Could you check a few things on this model? Use its own coordinates, in mm. A direction names the side the tool comes from. Give positions to 0.01 mm unless a question says otherwise; leave off trailing zeros. Write each loop counter-clockwise with the first axis right and the second up, starting at its lowest first coordinate (ties: lowest second). Pieces come first, ordered by that corner, then holes. Notation, with made-up numbers: (3, -14.75) -> (16, -14.75) arc R18 ccw to (16, 11.25) -> close; hole circle Ø10 at (-18, 57). An arc over 180 degrees is marked (long way). One line per question, with ' | ' between items.
from build123d import *

# Parameters (mm, degrees)
F0_R     = 6.5
F1_DEPTH = 2.5
F3_DEPTH = 9.6


# Not quite as in the source:
# - a feature of the source that left no trace in its solid (it failed there, or was rolled back) is left out


with BuildPart() as f1:
    # F0 (on Top) → F1 (new body)
    with BuildSketch(Plane.XY):
        Polygon((-30.6198447943, 27.4039022624), (-27.4521095872, 27.4039022624), (-8.6198447943, 27.4039022624), (-8.6198447943, 35.4039022624), (-13.1198447943, 35.4039022624), (-13.1198447943, 42.8039022624), (-22.6198447943, 42.8039022624), (-22.6198447943, 46.4039022624), (-30.6198447943, 46.4039022624), align=None)
        Polygon((-3.2843746781, 35.4039022624), (-3.2843746781, 27.4039022624), (15.5478901148, 27.4039022624), (18.7156253219, 27.4039022624), (18.7156253219, 46.4039022624), (10.7156253219, 46.4039022624), (10.7156253219, 42.8039022624), (1.2156253219, 42.8039022624), (1.2156253219, 35.4039022624), align=None)
        Polygon((-8.6198447943, 27.4039022624), (-27.4521095872, 27.4039022624), (-27.4521095872, -26.3960977376), (-6.0521095872, -26.3960977376), (-5.8521098852, -26.3960977376), (15.5478901148, -26.3960977376), (15.5478901148, 27.4039022624), (-3.2843746781, 27.4039022624), (-5.8521098852, 27.4039022624), (-6.0521095872, 27.4039022624), align=None)
        Polygon((-23.4521095872, -22.3960977376), (-23.4521095872, 23.4039022624), (-5.9521097362, 23.4039022624), (11.5478901148, 23.4039022624), (11.5478901148, -22.3960977376), (-5.9521097362, -22.3960977376), align=None, mode=Mode.SUBTRACT)
        Polygon((-5.9521097362, 23.4039022624), (-23.4521095872, 23.4039022624), (-23.4521095872, -22.3960977376), (-5.9521097362, -22.3960977376), (11.5478901148, -22.3960977376), (11.5478901148, 23.4039022624), align=None)
        with Locations((-5.9521097362, 0.5039022624)):
            Circle(F0_R, mode=Mode.SUBTRACT)
    extrude(amount=-F1_DEPTH)

    # F0 (on Top) → F3 (join)
    with BuildSketch(Plane.XY):
        Polygon((-8.6198447943, 27.4039022624), (-27.4521095872, 27.4039022624), (-27.4521095872, -26.3960977376), (-6.0521095872, -26.3960977376), (-5.8521098852, -26.3960977376), (15.5478901148, -26.3960977376), (15.5478901148, 27.4039022624), (-3.2843746781, 27.4039022624), (-5.8521098852, 27.4039022624), (-6.0521095872, 27.4039022624), align=None)
        Polygon((-23.4521095872, -22.3960977376), (-23.4521095872, 23.4039022624), (-5.9521097362, 23.4039022624), (11.5478901148, 23.4039022624), (11.5478901148, -22.3960977376), (-5.9521097362, -22.3960977376), align=None, mode=Mode.SUBTRACT)
    extrude(amount=F3_DEPTH)


solid = f1.part
Q1. Imagine slicing it at C-C on z = 5.25. Please give me the cut outline in (x, y), and give its area (3 significant figures).
Answer below:
outline: (-27.45, -26.4) -> (15.55, -26.4) -> (15.55, 27.4) -> (-27.45, 27.4) -> close; hole (-23.45, -22.4) -> (11.55, -22.4) -> (11.55, 23.4) -> (-23.45, 23.4) -> close | area: 710 mm^2
Q2. Imagine slicing it at B-B on x = -1.5. Please give me the cut outline in (y, z), and give its area (3 significant figures).
Answer below:
outline: (-26.4, -2.5) -> (-4.23, -2.5) -> (-4.23, 0) -> (-22.4, 0) -> (-22.4, 9.6) -> (-26.4, 9.6) -> close; (5.24, -2.5) -> (35.4, -2.5) -> (35.4, 0) -> (27.4, 0) -> (27.4, 9.6) -> (23.4, 9.6) -> (23.4, 0) -> (5.24, 0) -> close | area: 208 mm^2
Q3. Will these pins go through, and if not, where does the flat tip stop? pin 1 (0.8 mm diameter, centred on x = -17, z = -1.5, fed in from +Y); pin 2 (0.8 mm diameter, centred on x = -29.5, z = -1.5, fed in from -Y); pin 3 (9.5 mm diameter, centred on x = -20, y = 34.5, fed in from +Z); pin 4 (2 mm diameter, centred on x = -22.5, y = 13.5, fed in from +Z).
Answer below:
pin 1: stops at y = 42.8 | pin 2: stops at y = 27.4 | pin 3: stops at z = 0 | pin 4: stops at z = 9.6
Q4. On a 3-axis mill with a long thin cutter (end or side, diameter ignored), from which of +Z, -Z, +X, -X, +Y, -Y can I reach the whole of each face in a straight line? I mean faces 5 (the flat face through (-8.62, 31, -1)), 6 (the flat face through (-6, -22.396, 5)), 7 (the flat face through (-27.452, 1, 3)). Say none if no direction works.
Answer below:
face 5: +Z, -Z, +Y | face 6: +Z | face 7: +Z, -Z, -X, -Y
Q5. Imagine slicing it at A-A on y = 29. Please give me the cut outline in (x, z), and give its area (3 significant figures).
Answer below:
outline: (-30.62, -2.5) -> (-8.62, -2.5) -> (-8.62, 0) -> (-30.62, 0) -> close; (-3.28, -2.5) -> (18.72, -2.5) -> (18.72, 0) -> (-3.28, 0) -> close | area: 110 mm^2
Q6. Imagine slicing it at D-D on x = 8.5. Please give me the cut outline in (y, z), and give its area (3 significant figures).
Answer below:
outline: (-26.4, -2.5) -> (42.8, -2.5) -> (42.8, 0) -> (27.4, 0) -> (27.4, 9.6) -> (23.4, 9.6) -> (23.4, 0) -> (-22.4, 0) -> (-22.4, 9.6) -> (-26.4, 9.6) -> close | area: 250 mm^2
Q7. If I drill on line 1 along X through (y, z) = (-17, 0.5); line 2 along Y through (x, z) = (3, 8.25); line 3 along Y through (x, z) = (-5.5, -1.5), over which ranges is the centre line in solid material (lowest first)?
Answer below:
line 1: x = -27.45 to -23.45, 11.55 to 15.55 | line 2: y = -26.4 to -22.4, 23.4 to 27.4 | line 3: y = -26.4 to -5.98, 6.99 to 27.4
Q8. If we mould it in two halves opening along Y, with no side actions, what happens to faces 1 (the flat face through (15, 46.404, -1)), 2 (the flat face through (-22, 35, 0)), 3 (the flat face through (-6, 23.404, 5)), 4 (the cylindrical face through (0.248, 2.456, -1.232))? For each: +Y half, -Y half, draft (parallel to the pull), parting line (faces both ways), or undercut.
Answer below:
face 1: +Y half | face 2: draft | face 3: undercut | face 4: undercut
